```python
from build123d import *

# Parameters (mm, degrees)
PAD_DEPTH    = 46
CHAMFER_SIZE = 0.7
FILLET_R     = 1
POCKET_DEPTH = 2


with BuildPart() as part:
    # Sketch → Pad (new body)
    with BuildSketch(Plane.XY):
        Polygon((-26.095954, 27.107406), (35.904046, 27.107406), (35.904046, 24.807406), (38.204046, 24.807406), (38.204046, 23.307406), (34.404046, 23.307406), (34.404046, 25.607406), (-24.595954, 25.607406), (-24.595954, 23.307406), (-28.395954, 23.307406), (-28.395954, 24.807406), (-26.095954, 24.807406), align=None)
    extrude(amount=PAD_DEPTH)

    # Chamfer
    chamfer_edges = [part.edges().sort_by_distance(p)[0] for p in [
        (35.904046, 27.107406, 23),
        (-26.095954, 27.107406, 23),
    ]]
    chamfer(chamfer_edges, length=CHAMFER_SIZE)

    # Fillet
    fillet_edges = [part.edges().sort_by_distance(p)[0] for p in [
        (-24.595954, 23.307406, 23),
        (34.404046, 23.307406, 23),
    ]]
    fillet(fillet_edges, radius=FILLET_R)

    # Sketch001 (on Face12 of Fillet) → Pocket (cut)
    with BuildSketch(Plane(origin=(0, 27.107406, 0), x_dir=(-1, 0, 0), z_dir=(0, 1, 0))):
        with BuildLine():
            Line((20.895954, 25), (-7.104046, 25))
            ThreePointArc((-7.104046, 25), (-7.811153, 24.707107), (-8.104046, 24))
            Line((-8.104046, 24), (-8.104046, 11))
            ThreePointArc((-8.104046, 11), (-7.811153, 10.292893), (-7.104046, 10))
            Line((-7.104046, 10), (20.895954, 10))
            ThreePointArc((20.895954, 10), (21.603061, 10.292893), (21.895954, 11))
            Line((21.895954, 11), (21.895954, 24))
            ThreePointArc((21.895954, 24), (21.603061, 24.707107), (20.895954, 25))
        make_face()
    extrude(amount=-POCKET_DEPTH, mode=Mode.SUBTRACT)


solid = part.part
```
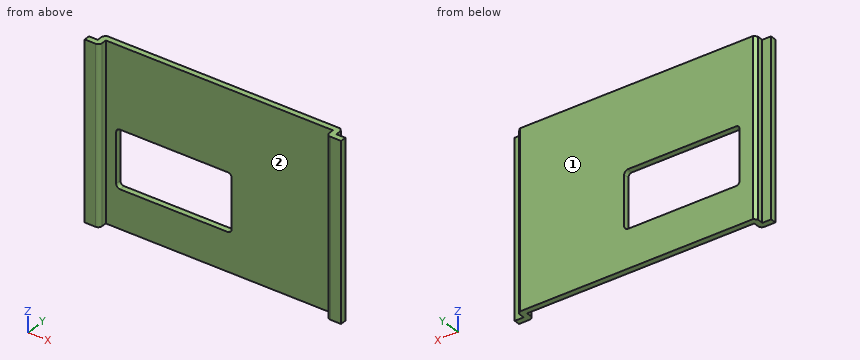
Part model, mm, in its own coordinate system. Face numbers are marked on the shaded views. Round coordinates to 2 decimals unless told otherwise and drop trailing zeros. Loops run counter-clockwise (first coordinate to the right, second up) from the corner with the lowest first, then second, coordinate; pieces in that order, holes last. Notation, with made-up numbers: (43.5, 69) -> (81.5, 69) arc R27 ccw to (81.5, 105) -> close; hole circle Ø5 at (59.5, 0.5). An arc over 180 degrees is marked (long way). Use CSV: the item, a comma, the result in double quotes. Start each with the question number.
1) Drop flat-ended pins along their axis: P1, Ø5, axis at x = 23, z = 27, coming from the -Y side; P2, Ø1.6, axis at y = 26, z = 19.5, coming from the +X side; P3, Ø0.7, axis at x = 36.5, z = 22, coming from the +Y side. Give the stop position or say it passes through.
2) Cut at B-B, the plane x = -13.5. Write the cut outline in (y, z).
3) Pull direction X, two halves, no side cores. Call the marked faces 1 and 2: +X half, -X half, draft (parallel to the pull), parting line (faces both ways), or undercut.
4) Cut at C-C, the plane z = 30. Write the cut outline in (x, y), plus the area to 3 significant figures.
5) Cut at A-A, the plane z = 12. Write the cut outline in (x, y), plus the area to 3 significant figures.
6) Cut at D-D, the plane x = 26. Write the cut outline in (y, z), plus the area to 3 significant figures.
7) Wall check: L1, parallel to Z at x = -11, y = 26.6; L2, parallel to X at y = 25.3, z = 19.5; L3, parallel to X at y = 24.35, z = 40. Give the ranges that are in metal, low to high. Write a range as [from, to].
Determined:
1,P1,"stops at y = 25.61"
1,P2,"stops at x = 35.9"
1,P3,"stops at y = 24.81"
2,outline,"(25.61, 0) -> (27.11, 0) -> (27.11, 10) -> (25.61, 10) -> close; (25.61, 25) -> (27.11, 25) -> (27.11, 46) -> (25.61, 46) -> close"
3,face 1,"draft"
3,face 2,"undercut"
4,outline,"(-28.4, 23.31) -> (-25.6, 23.31) arc R1 ccw to (-24.6, 24.31) -> (-24.6, 25.61) -> (34.4, 25.61) -> (34.4, 24.31) arc R1 ccw to (35.4, 23.31) -> (38.2, 23.31) -> (38.2, 24.81) -> (35.9, 24.81) -> (35.9, 26.41) -> (35.2, 27.11) -> (-25.4, 27.11) -> (-26.1, 26.41) -> (-26.1, 24.81) -> (-28.4, 24.81) -> close"
4,area,"106 mm2"
5,outline,"(-28.4, 23.31) -> (-25.6, 23.31) arc R1 ccw to (-24.6, 24.31) -> (-24.6, 25.61) -> (-21.9, 25.61) -> (-21.9, 27.11) -> (-25.4, 27.11) -> (-26.1, 26.41) -> (-26.1, 24.81) -> (-28.4, 24.81) -> close; (8.1, 25.61) -> (34.4, 25.61) -> (34.4, 24.31) arc R1 ccw to (35.4, 23.31) -> (38.2, 23.31) -> (38.2, 24.81) -> (35.9, 24.81) -> (35.9, 26.41) -> (35.2, 27.11) -> (8.1, 27.11) -> close"
5,area,"60.9 mm2"
6,outline,"(25.61, 0) -> (27.11, 0) -> (27.11, 46) -> (25.61, 46) -> close"
6,area,"69.0 mm2"
7,L1,"z = [0, 10], [25, 46]"
7,L2,"x = [-26.1, -24.6], [34.4, 35.9]"
7,L3,"x = [-28.4, -24.6], [34.4, 38.2]"
